Model file for the job. Use its own axes, mm. Round coordinates to 2 decimals unless told otherwise and drop trailing zeros. Order: outer loops, then holes, each group sorted by start corner. A loop starts at its lowest first (then second) coordinate and runs counter-clockwise, first axis right, second up. Notation, with made-up numbers: (83.5, 1) -> (122.5, 1) arc R36 ccw to (122.5, 39) -> close; hole circle Ø7 at (43, 60). An arc over 180 degrees is marked (long way). Put each result on its own line as item: value. Start each with the question number.
Q1. Cut at C-C, the plane z = 4.25. List the corners of the cut face in (x, y).
Q2. Probe L1, parallel to Z at x = -38.5, y = -101.5; L2, parallel to Z at x = -1, y = -121; L3, parallel to X at y = -131.5, z = -3.25. List the from-to ranges inside material, lowest first.
Q3. Cut at B-B, the plane x = 19. List the corners of the cut face in (y, z).
Q4. Cut at A-A, the plane y = -100. List the corners of the cut face in (x, z), and give its area (3 significant figures).
Q5. Flat gauge pins, fed straight in: P1, Ø1.5, axis at x = -49, y = -16, coming from the +Z side; P2, Ø1.5, axis at y = -119, z = -2, coming from the +X side; P3, Ø10, axis at y = -82.5, z = 2, coming from the +X side. Where does each tip first touch, or does it go through?
from build123d import *

# Parameters (mm, degrees)
F1_DEPTH = 150
F2_R     = 5


with BuildPart() as f1:
    # F0 (on Front) → F1 (new body)
    with BuildSketch(Plane.XZ):
        with BuildLine():
            Line((-82.3190790229, 12.2144147383), (-82.3190790229, -7.7855852617))
            Line((-82.3190790229, -7.7855852617), (47.6809209771, -7.7855852617))
            ThreePointArc((47.6809209771, -7.7855852617), (45.7765227323, -3.9495345355), (41.9135876, -2.1002779249))
            Line((41.9135876, -2.1002779249), (-82.3190790229, 12.2144147383))
        make_face()
    extrude(amount=F1_DEPTH)

    # F2
    f2_edges = [f1.edges().sort_by_distance(p)[0] for p in [
        (-82.319079, -75, 12.214415),
        (-82.319079, -75, -7.785585),
    ]]
    fillet(f2_edges, radius=F2_R)


solid = f1.part
Ans:
1. outline: (-82.32, -150) -> (-13.2, -150) -> (-13.2, 0) -> (-82.32, 0) -> close
2. L1: z = -7.79 to 7.17
2. L2: z = -7.79 to 2.84
2. L3: x = -82.3 to 44.94
3. outline: (-150, -7.79) -> (0, -7.79) -> (0, 0.54) -> (-150, 0.54) -> close
4. outline: (-82.32, -2.79) arc R5 ccw to (-77.32, -7.79) -> (47.68, -7.79) arc R6.57 ccw to (41.91, -2.1) -> (-76.75, 11.57) arc R5 ccw to (-82.32, 6.61) -> close
4. area: 1,610 mm^2
5. P1: stops at z = 8.46
5. P2: stops at x = 44.1
5. P3: stops at x = 44.55
